Geometry check sheet. Reference: the model listing, model coordinates, mm. Round coordinates to 2 decimals unless told otherwise and drop trailing zeros. Write each loop counter-clockwise with the first axis right and the second up, starting at its lowest first coordinate (ties: lowest second). Pieces come first, ordered by that corner, then holes.
Autodesk Inventor part; units mm, degrees
ref_plane "YZ Plane" through (0, 0, 0) normal (1, 0, 0) x (0, 1, 0)
ref_plane "XZ Plane" through (0, 0, 0) normal (0, 1, 0) x (-1, 0, 0)
ref_plane "XY Plane" through (0, 0, 0) normal (0, 0, 1) x (1, 0, 0)
sketch "Skizze1" plane through (0, 0, 0) normal (0, 0, 1) x (1, 0, 0)
  circle A0 centre (0, 0) radius 15
  circle A1 centre (0, 0) radius 11.1
  dimension "d0" = 30
  dimension "d1" = 22.2
extrude "Extrusion1" add sketch "Skizze1" along normal blind 20
sketch "Skizze2" plane through (0, 0, 20) normal (0, 0, 1) x (1, 0, 0)
  circle A0 centre (0, 0) radius 15
  circle A1 centre (0, 0) radius 11.1
  circle A2 centre (0, 0) radius 26.2393
  circle A3 centre (0, 0) radius 15
extrude "Extrusion2" add sketch "Skizze2" against normal blind 5 contours A2
sketch "Skizze3" plane through (0, 0, 20) normal (0, 0, 1) x (1, 0, 0)
  circle A0 centre (0, 0) radius 26.2393
  line L0 (-36.7351, 0) -> (36.7351, 0)
  line L1 (0, -36.7351) -> (0, 36.7351)
  point P0 (0, 20)
  point P1 (-20, 0)
  point P2 (0, -20)
  point P3 (20, 0)
  dimension "d6" = 20
  dimension "d7" = 20
  dimension "d8" = 20
  dimension "d9" = 20
hole "Bohrung1" at (0, 20, 20) at (-20, 0, 20) at (0, -20, 20) at (20, 0, 20) direction (0, 0, -1) diameter 4.4 end through all
properties part number "Cameralager21.8"
1. Section check B-B (y = 20). Record the cut outline in (x, z), plus the area to 3 significant figures.
2. Release check for a two-part mould opening along X. For faces 1 (the face through (0.843, 17.968, 17.465)), 2 (the face through (11, -11, 15)), 3 (the face through (-14.985, -0.66, 7.395)) record: +X half, -X half, draft (parallel to the pull), parting line (faces both ways), or undercut.
3. Depth check by flat-ended pin: pin 1 Ø10 at (x, z) = (8.5, 14) entering from -Y; pin 2 Ø10 at (y, z) = (10, 9) entering from +X; pin 3 Ø5 at (x, z) = (-13, 10.5) entering from -Y. Enter the tip coordinate at first touch or a pass-through.
4. Section check A-A (x = 0). Record the cut outline in (y, z).
5. Scan lines: line 1 along Y through (x, z) = (0, 17); line 2 along Y through (x, z) = (-0.5, 17.75); line 3 along Y through (x, z) = (3.5, 17). Record each from-to range of solid material in increasing order.
6. Section check C-C (z = 3.75). Record the cut outline in (x, y).
7. Section check D-D (x = 19). Record the cut outline in (y, z).
Results below:
1. outline: (-16.99, 15) - (-2.2, 15) - (-2.2, 20) - (-16.99, 20) - close; (2.2, 15) - (16.99, 15) - (16.99, 20) - (2.2, 20) - close
1. area: 148 mm2
2. face 1: undercut
2. face 2: draft
2. face 3: parting line
3. pin 1: stops at y = -25.99
3. pin 2: stops at x = 14.14
3. pin 3: stops at y = -10.71
4. outline: (-26.24, 15) - (-22.2, 15) - (-22.2, 20) - (-26.24, 20) - close; (-17.8, 15) - (-15, 15) - (-15, 0) - (-11.1, 0) - (-11.1, 20) - (-17.8, 20) - close; (11.1, 0) - (15, 0) - (15, 15) - (17.8, 15) - (17.8, 20) - (11.1, 20) - close; (22.2, 15) - (26.24, 15) - (26.24, 20) - (22.2, 20) - close
5. line 1: y = -26.24 to -22.2, -17.8 to -11.1, 11.1 to 17.8, 22.2 to 26.24
5. line 2: y = -26.23 to -22.14, -17.86 to -11.09, 11.09 to 17.86, 22.14 to 26.23
5. line 3: y = -26 to -10.53, 10.53 to 26
6. outline: circle Ø30 at (0, 0); hole circle Ø22.2 at (0, 0)
7. outline: (-18.1, 15) - (-1.96, 15) - (-1.96, 20) - (-18.1, 20) - close; (1.96, 15) - (18.1, 15) - (18.1, 20) - (1.96, 20) - close
